Autodesk Inventor part; units mm, degrees
ref_plane "YZ Plane" through (0, 0, 0) normal (1, 0, 0) x (0, 1, 0)
ref_plane "XZ Plane" through (0, 0, 0) normal (0, 1, 0) x (-1, 0, 0)
ref_plane "XY Plane" through (0, 0, 0) normal (0, 0, 1) x (1, 0, 0)
sketch "Sketch5" plane through (0, 0, 0) normal (0, 0, 1) x (1, 0, 0)
  line L0 (0, 0) -> (0, 60)
  line L1 (0, 0) -> (10, 0)
  line L2 (10, 0) -> (10, 7)
  line L3 (10, 7) -> (15.85, 7)
  line L4 (15.85, 7) -> (15.85, 11)
  line L5 (15.85, 11) -> (10, 11)
  line L6 (10, 11) -> (10, 27)
  line L7 (10, 27) -> (15.85, 27)
  line L8 (15.85, 31) -> (10, 31)
  line L9 (10, 31) -> (10, 60)
  line L10 (10, 60) -> (0, 60)
  line L11 (15.85, 31) -> (15.85, 27)
  dimension "d17" = 31.7
  dimension "d18" = 7
  dimension "d19" = 4
  dimension "d23" = 20
  dimension "d26" = 60
  dimension "d27" = 20
  dimension "d48" = 31.7
  dimension "d49" = 16
  dimension "d50" = 4
revolve "Revolution1" add sketch "Sketch5" angle 360 about axis through (0, 0, 0) along (0, 1, 0)
sketch "Sketch6" plane through (0, 0, 0) normal (0, -1, 0) x (1, 0, 0)
  line L0 (-6, 0) -> (6, 0)
  circle A0 centre (0, 6) radius 4
  point P0 (0, 0)
  point P1 (6, 0)
  point P2 (0, 0)
  dimension "d29" = 12
  dimension "d56" = 8
  dimension "d57" = 6
hole "Hole2" at (6, 0, 0) at (-6, 0, 0) at (0, 0, 6) direction (0, 1, 0) diameter 3 end through all counterbore diameter 5 counterbore depth 15
sketch "Sketch8" plane through (0, 7, 0) normal (0, -1, 0) x (1, 0, 0)
  line L0 (-17.88, 0) -> (-13.88, 0) construction
  line L1 (-17.88, 1.5) -> (-13.88, 1.5)
  line L2 (-13.88, -1.5) -> (-17.88, -1.5)
  arc A0 (-17.88, 1.5) -> (-17.88, -1.5) centre (-17.88, 0) ccw
  arc A1 (-13.88, -1.5) -> (-13.88, 1.5) centre (-13.88, 0) ccw
  point P0 (0, 0)
  point P1 (-15.88, 0)
  dimension "d40" = 13.88
  dimension "d41" = 1.5
  dimension "d42" = 4
extrude "Extrusion5" cut sketch "Sketch8" against normal up to surface (4 mm away)
pattern_circular "Circular Pattern1" count 4 over 360 about axis through (0, 3.5, 0) along (0, 1, 0) of "Extrusion5"
sketch "Sketch9" plane through (0, 60, 0) normal (0, 1, 0) x (1, 0, 0)
  circle A0 centre (-6, 0) radius 1.5
  circle A1 centre (6, 0) radius 1.5
  circle A2 centre (-6, 0) radius 2.5
  circle A3 centre (6, 0) radius 1.5
  circle A4 centre (6, 0) radius 2.5
  circle A5 centre (0, -6) radius 1.5
  circle A6 centre (0, -6) radius 1.5
  circle A7 centre (0, -6) radius 2.5
  point P0 (0, 0)
  point P1 (0, 0)
  dimension "d51" = 5
  dimension "d53" = 5
  dimension "d68" = 5
extrude "Extrusion6" cut sketch "Sketch9" against normal blind 15 contours A2 | A4 | A5 | A7
sketch "Sketch10" plane through (0, 0, 0) normal (0, -1, 0) x (1, 0, 0)
  point P0 (0, 0)
  point P1 (0, 0)
hole "Hole3" at (0, 0, 0) direction (0, 1, 0) diameter 3 depth 10 tip angle 118
sketch "Sketch11" plane through (0, 0, 0) normal (0, -1, 0) x (1, 0, 0)
  circle A0 centre (0, 6) radius 2.5
  line L0 (0, 6) -> (0, 17) construction
  line L1 (-2.5, 6) -> (-2.5, 17)
  line L2 (2.5, 17) -> (2.5, 6)
  arc A1 (-2.5, 6) -> (2.5, 6) centre (0, 6) ccw
  arc A2 (2.5, 17) -> (-2.5, 17) centre (0, 17) ccw
  point P0 (0, 0)
  point P1 (0, 11.5)
  point P2 (-2.5, 6)
  point P3 (2.5, 6)
  dimension "d65" = 11
extrude "Extrusion7" cut sketch "Sketch11" against normal blind 7.5 contours A0 L1 A2 L2
properties part number "033" material "Glass"
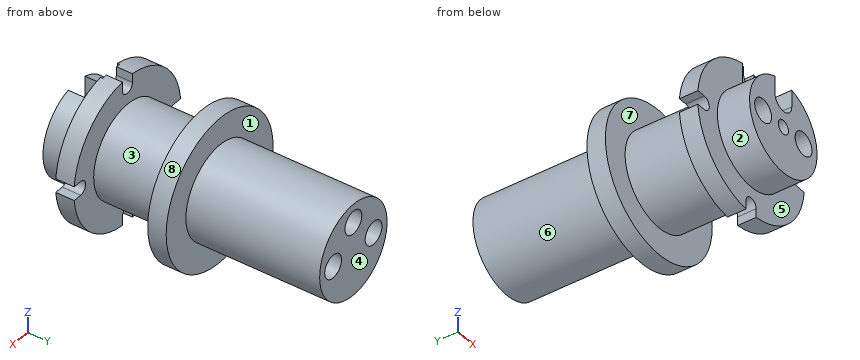
Geometry: final body of the model. Coordinates: model frame, mm. Face numbers are marked on the shaded views. A direction names the side the tool comes from. Round coordinates to 2 decimals unless told otherwise and drop trailing zeros. Loops run counter-clockwise (first coordinate to the right, second up) from the corner with the lowest first, then second, coordinate; pieces in that order, holes last. Notation, with made-up numbers: (34.5, 79.25) -> (74.5, 79.25) arc R26 ccw to (74.5, 96.25) -> close; hole circle Ø9 at (22, -37). An arc over 180 degrees is marked (long way). Use one line per item in the form item = value.
Item 1: Cut plane A-A on y = 9. Output: boundary loops of the cut face in (x, z).
Evaluation:
outline = (-15.78, -1.5) arc R15.85 ccw to (-1.5, -15.78) -> (-1.5, -13.88) arc R1.5 cw to (1.5, -13.88) -> (1.5, -15.78) arc R15.85 ccw to (15.78, -1.5) -> (13.88, -1.5) arc R1.5 cw to (13.88, 1.5) -> (15.78, 1.5) arc R15.85 ccw to (1.5, 15.78) -> (1.5, 13.88) arc R1.5 cw to (-1.5, 13.88) -> (-1.5, 15.78) arc R15.85 ccw to (-15.78, 1.5) -> (-13.88, 1.5) arc R1.5 cw to (-13.88, -1.5) -> close; hole circle Ø5 at (-6, 0); hole circle Ø5 at (0, 6); hole circle Ø3 at (0, 0); hole circle Ø5 at (6, 0)
Item 2: Cut plane C-C on y = 48.5. Output: boundary loops of the cut face in (x, z).
Evaluation:
outline = circle Ø20 at (0, 0); hole circle Ø5 at (-6, 0); hole circle Ø5 at (0, 6); hole circle Ø5 at (6, 0)
Item 3: Cut plane B-B on z = -11. Output: boundary loops of the cut face in (x, y), then the cut area to 3 significant figures.
Evaluation:
outline = (-11.41, 7) -> (11.41, 7) -> (11.41, 11) -> (-11.41, 11) -> close; (-11.41, 27) -> (11.41, 27) -> (11.41, 31) -> (-11.41, 31) -> close
area = 183 mm2
Item 4: Access query for the marked faces 4, 5, 6, 7 and 8. Directions: +Z, -Z, +X, -X, +Y, -Y. A direction counts if a zero-diameter tool reaches every point of the face in a straight line with its end or side. Return the directions, or none.
Evaluation:
face_4 = +Z, -Z, +X, -X, +Y
face_5 = -Y
face_6 = +Y
face_7 = none
face_8 = +Y, -Y
Item 5: Material intervals for probe 1 along X at (y, z) = (48.5, 0); probe 2 along Z at (x, y) = (0, 38.25), sorted ascending.
Evaluation:
probe_1 = -10 to -8.5, -3.5 to 3.5, 8.5 to 10
probe_2 = -10 to 4.5, 7.5 to 10
Item 6: Contact query for flat-ended pins moving along their axis: pin 1 Ø8 at (y, z) = (17, -5.5) entering from +X; pin 2 Ø1.5 at (y, z) = (9, 15) entering from +X; pin 3 Ø12 at (y, z) = (9, 5.5) entering from -X. Output: stop coordinate, or through.
Evaluation:
pin_1 = 9.89
pin_2 = 6.94
pin_3 = -15.78
Item 7: Cut plane D-D on z = -5. Output: boundary loops of the cut face in (x, y), then the cut area to 3 significant figures.
Evaluation:
outline = (-15.04, 7) -> (-8.66, 7) -> (-8.66, 0) -> (8.66, 0) -> (8.66, 7) -> (15.04, 7) -> (15.04, 11) -> (8.66, 11) -> (8.66, 27) -> (15.04, 27) -> (15.04, 31) -> (8.66, 31) -> (8.66, 60) -> (-8.66, 60) -> (-8.66, 31) -> (-15.04, 31) -> (-15.04, 27) -> (-8.66, 27) -> (-8.66, 11) -> (-15.04, 11) -> close
area = 1,140 mm2
Item 8: Draft query along Y for the marked faces 1, 2 and 3. Return one class per face: released by +Y, released by -Y, zero draft, split by the parting line, or undercut.
Evaluation:
face_1 = released by +Y
face_2 = zero draft
face_3 = undercut
